The listing builds one solid part. Answer for the finished solid, in the listing's coordinates (mm). Face numbers are marked on the shaded views. A direction names the side the tool comes from. Give positions to 0.01 mm unless a question says otherwise; leave off trailing zeros. Order: outer loops, then holes, each group sorted by start corner. A loop starts at its lowest first (then second) coordinate and runs counter-clockwise, first axis right, second up. Notation, with made-up numbers: (-33.5, 41.25) - (9.5, 41.25) arc R18 cw to (9.5, 68.25) - close; hole circle Ø10 at (58.25, 69). An arc over 180 degrees is marked (long way). Answer in a Markdown table with one row per item.
from build123d import *

# Parameters (mm, degrees)
F1_DEPTH  = 50.8
F2_DEPTH  = 6.35
F3_R      = 3.81
F4_DEPTH  = 19.05
F5_R      = 6.35
F6_DEPTH  = 6.35
F7_R      = 2.54
F8_DEPTH  = 12.701
F9_R      = 2.54
F10_DEPTH = 81.281
F9_R_2    = 6.35
F11_DEPTH = 68.58


with BuildPart() as f1:
    # F0 (on Front) → F1 (new body)
    with BuildSketch(Plane.XZ):
        with BuildLine():
            Line((0, 50.8), (0, 0))
            Line((0, 0), (-43.18, 0))
            Line((-43.18, 0), (-43.18, 50.8))
            Line((-43.18, 50.8), (-46.99, 50.8))
            ThreePointArc((-46.99, 50.8), (-57.766307, 46.336307), (-62.23, 35.56))
            Line((-62.23, 35.56), (-62.23, 0))
            ThreePointArc((-62.23, 0), (-43.631281, -44.901281), (1.27, -63.5))
            Line((1.27, -63.5), (19.05, -63.5))
            Line((19.05, -63.5), (19.05, 50.8))
            Line((19.05, 50.8), (0, 50.8))
        make_face()
    extrude(amount=F1_DEPTH)

    # F0 (on Front) → F2 (join)
    with BuildSketch(Plane.XZ):
        Polygon((-43.18, 0), (0, 0), (0, 50.8), (-12.7, 50.8), (-12.7, 12.7), (-30.48, 12.7), (-30.48, 50.8), (-43.18, 50.8), align=None)
        with BuildLine():
            Line((0, 50.8), (0, 0))
            Line((0, 0), (-43.18, 0))
            Line((-43.18, 0), (-43.18, 50.8))
            Line((-43.18, 50.8), (-46.99, 50.8))
            ThreePointArc((-46.99, 50.8), (-57.766307, 46.336307), (-62.23, 35.56))
            Line((-62.23, 35.56), (-62.23, 0))
            ThreePointArc((-62.23, 0), (-43.631281, -44.901281), (1.27, -63.5))
            Line((1.27, -63.5), (19.05, -63.5))
            Line((19.05, -63.5), (19.05, 50.8))
            Line((19.05, 50.8), (0, 50.8))
        make_face()
    extrude(amount=F2_DEPTH)

    # F3 (on face) → F4 (cut, through all)
    with BuildSketch(Plane(origin=(-62.23, 0, 0), x_dir=(0, -1, 0), z_dir=(-1, 0, 0))):
        with Locations((25.4, 25.4)):
            Circle(F3_R)
    extrude(amount=-F4_DEPTH, mode=Mode.SUBTRACT)

    # F5 (on face) → F6 (cut)
    with BuildSketch(Plane(origin=(0, 0, 0), x_dir=(0, -1, 0), z_dir=(-1, 0, 0))):
        with Locations((25.4, 25.4)):
            Circle(F5_R)
    extrude(amount=-F6_DEPTH, mode=Mode.SUBTRACT)

    # F7 (on face) → F8 (cut, through all)
    with BuildSketch(Plane(origin=(6.35, 0, 0), x_dir=(0, -1, 0), z_dir=(-1, 0, 0))):
        with Locations((25.4, 25.4)):
            Circle(F7_R)
    extrude(amount=-F8_DEPTH, mode=Mode.SUBTRACT)

    # F9 (on face) → F10 (cut, through all)
    with BuildSketch(Plane(origin=(-62.23, 0, 0), x_dir=(0, -1, 0), z_dir=(-1, 0, 0))):
        with Locations((25.4, -38.1)):
            Circle(F9_R)
    extrude(amount=-F10_DEPTH, mode=Mode.SUBTRACT)

    # F9 (on face) → F11 (cut)
    with BuildSketch(Plane(origin=(-62.23, 0, 0), x_dir=(0, -1, 0), z_dir=(-1, 0, 0))):
        with Locations((25.4, -38.1)):
            Circle(F9_R_2)
        with Locations((25.4, -38.1)):
            Circle(F9_R, mode=Mode.SUBTRACT)
    extrude(amount=-F11_DEPTH, mode=Mode.SUBTRACT)


solid = f1.part
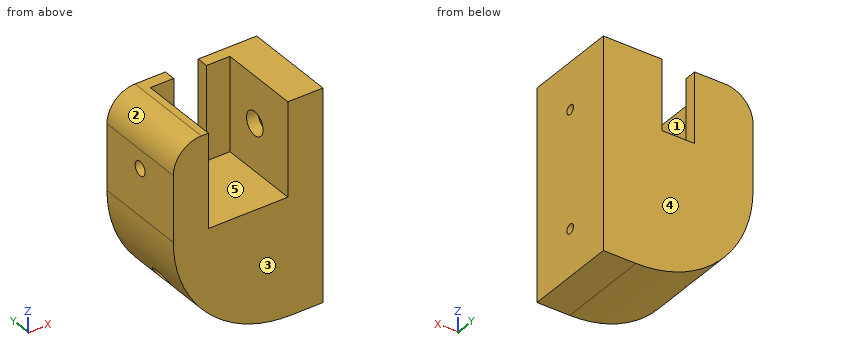
Item 1: Each of these flat-tipped pins is pushed along its axis until it touches: P1, Ø16.5, axis at y = -25.4, z = 25.4, coming from the -X side; P2, Ø10, axis at y = -26, z = -35, coming from the -X side; P3, Ø21.5, axis at x = -15.5, y = -33.5, coming from the +Z side; P4, Ø3, axis at y = -39, z = -21, coming from the -X side. Where does it stop, or does it pass through?
Answer block:
| item | result |
|---|---|
| P1 | x = -62.23 |
| P2 | x = -54.7 |
| P3 | z = 0 |
| P4 | x = -59.16 |
Item 2: Find section C-C on x = -34.5. Write down the section's boundary in (y, z).
Answer block:
| item | result |
|---|---|
| outline | (-50.8, -52.47) - (0, -52.47) - (0, 50.8) - (-6.35, 50.8) - (-6.35, 0) - (-50.8, 0) - close; hole circle Ø12.7 at (-25.4, -38.1) |
Item 3: Find section D-D on z = -38.1. Write down the section's boundary in (x, y), then the cut area to 3 significant figures.
Answer block:
| item | result |
|---|---|
| outline | (-49.53, -50.8) - (19.05, -50.8) - (19.05, -27.94) - (6.35, -27.94) - (6.35, -31.75) - (-49.53, -31.75) - close; (-49.53, -19.05) - (6.35, -19.05) - (6.35, -22.86) - (19.05, -22.86) - (19.05, 0) - (-49.53, 0) - close |
| area | 2,710 mm² |
Item 4: Find section B-B on y = -25.4. Count the separate pieces of the cut face and the enclosed holes in it, then the cut area to 3 significant figures.
Answer block:
| item | result |
|---|---|
| separate pieces | 4 |
| enclosed holes | 0 |
| area | 5,120 mm² |
Item 5: Which of the six approach directions +Z, -Z, +X, -X, +Y, -Y give full straight-line access (tool end or side, diameter ignored) to the marked faces 4 and 5?
Answer block:
| item | result |
|---|---|
| face 4 | +Z, -Z, +X, -X, +Y |
| face 5 | +Z, -Y |
Item 6: Determine the mould class of the marked faces 1, 2 and 3 for opening direction X: pulls with the +X half, pulls with the -X half, needs draft (parallel to the pull), parting line crosses it, or undercut.
Answer block:
| item | result |
|---|---|
| face 1 | undercut |
| face 2 | pulls with the -X half |
| face 3 | needs draft |
Item 7: Find section A-A on z = 25.4. Write down the section's boundary in (x, y), then the cut area to 3 significant figures.
Answer block:
| item | result |
|---|---|
| outline | (-62.23, -50.8) - (-43.18, -50.8) - (-43.18, -29.21) - (-62.23, -29.21) - close; (-62.23, -21.59) - (-43.18, -21.59) - (-43.18, -6.35) - (-30.48, -6.35) - (-30.48, 0) - (-62.23, 0) - close; (-12.7, -6.35) - (0, -6.35) - (0, -19.05) - (6.35, -19.05) - (6.35, -22.86) - (19.05, -22.86) - (19.05, 0) - (-12.7, 0) - close; (0, -50.8) - (19.05, -50.8) - (19.05, -27.94) - (6.35, -27.94) - (6.35, -31.75) - (0, -31.75) - close |
| area | 1,810 mm² |
Item 8: Consider line 1 (X direction, y = -4, z = 30.5); line 2 (X direction, y = -24.5, z = 17); line 3 (Y direction, x = -34, z = -38.1). Determine where each line is inside the solid, lowest interval first.
Answer block:
| item | result |
|---|---|
| line 1 | -62.23 to -30.48, -12.7 to 19.05 |
| line 2 | -62.23 to -43.18, 0 to 19.05 |
| line 3 | -50.8 to -31.75, -19.05 to 0 |
